Here's how the part is built. I have some questions about the finished solid (model axes, mm). Face numbers are marked on the shaded views. Round coordinates to 2 decimals unless told otherwise and drop trailing zeros. Write each loop counter-clockwise with the first axis right and the second up, starting at its lowest first coordinate (ties: lowest second). Pieces come first, ordered by that corner, then holes. Notation, with made-up numbers: (-39.75, 78) -> (6.25, 78) arc R20 ccw to (6.25, 109) -> close; hole circle Ø1 at (38.25, -5.75). An arc over 180 degrees is marked (long way). Answer in a Markdown table with one row per item.
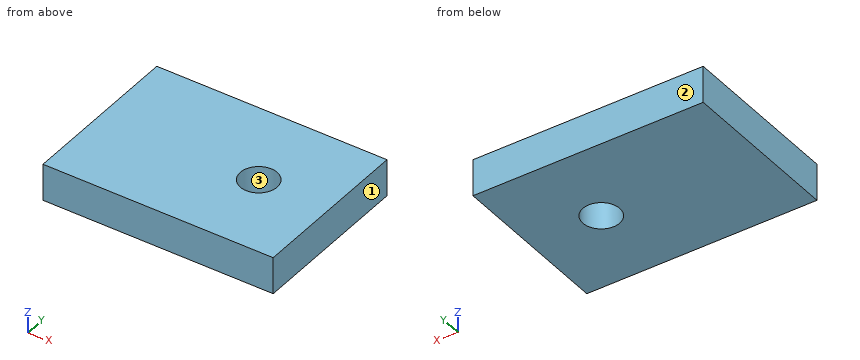
from build123d import *

# Parameters (mm, degrees)
SZKIC1_W                    = 25
SZKIC1_H                    = 18
DODANIE_WYCI_GNI_CIE1_DEPTH = 4
WYTNIJ_WYCI_GNI_CIE1_REACH  = 17.914
SZKIC2_R                    = 2


with BuildPart() as part:
    # Szkic1 → Dodanie-wyciągnięcie1 (new body)
    with BuildSketch(Plane.XY):
        Rectangle(SZKIC1_W, SZKIC1_H)
    extrude(amount=DODANIE_WYCI_GNI_CIE1_DEPTH)

    # Szkic2 → Wytnij-wyciągnięcie1 (cut, up to next)
    with BuildSketch(Plane.XY.offset(4), mode=Mode.PRIVATE) as wytnij_wyci_gni_cie1_sk1:
        with Locations((4.75, 0)):
            Circle(SZKIC2_R)
    wytnij_wyci_gni_cie1_tool1 = extrude(wytnij_wyci_gni_cie1_sk1.sketch, amount=-WYTNIJ_WYCI_GNI_CIE1_REACH, mode=Mode.PRIVATE) & part.part
    add(wytnij_wyci_gni_cie1_tool1.solids().sort_by_distance((4.75, 0, 4))[0], mode=Mode.SUBTRACT)


solid = part.part
1) I want a section at B-B, the plane y = 0. List the corners of the cut face in (x, z) for me.
Response:
| item | result |
|---|---|
| outline | (-12.5, 0) -> (2.75, 0) -> (2.75, 4) -> (-12.5, 4) -> close; (6.75, 0) -> (12.5, 0) -> (12.5, 4) -> (6.75, 4) -> close |
2) I need wall thicknesses on line 1 (Y direction, x = 4.75, z = 1.45); line 2 (X direction, y = -0.5, z = 3.2); line 3 (X direction, y = -0.75, z = 0.3). Which ranges of each line are inside material? Lowest first, please. Write a range as [from, to].
Response:
| item | result |
|---|---|
| line 1 | y = [-9, -2], [2, 9] |
| line 2 | x = [-12.5, 2.81], [6.69, 12.5] |
| line 3 | x = [-12.5, 2.9], [6.6, 12.5] |
3) I want a section at A-A, the plane x = 4.75. List the corners of the cut face in (y, z) for me.
Response:
| item | result |
|---|---|
| outline | (-9, 0) -> (-2, 0) -> (-2, 4) -> (-9, 4) -> close; (2, 0) -> (9, 0) -> (9, 4) -> (2, 4) -> close |
4) For pin 1 (2.5 mm diameter, centred on x = 4.75, y = 0, fed in from -Z), with a flat end and sliding along its axis, tell me the tip position at first contact or that it passes through.
Response:
| item | result |
|---|---|
| pin 1 | passes through |
5) We'd pull the mould along Y, two halves only. Please class the marked faces 1, 2 and 3: +Y half, -Y half, draft (parallel to the pull), parting line (faces both ways), or undercut.
Response:
| item | result |
|---|---|
| face 1 | draft |
| face 2 | +Y half |
| face 3 | undercut |
6) I want a section at C-C, the plane z = 1. List the corners of the cut face in (x, y) for me.
Response:
| item | result |
|---|---|
| outline | (-12.5, -9) -> (12.5, -9) -> (12.5, 9) -> (-12.5, 9) -> close; hole circle Ø4 at (4.75, 0) |
